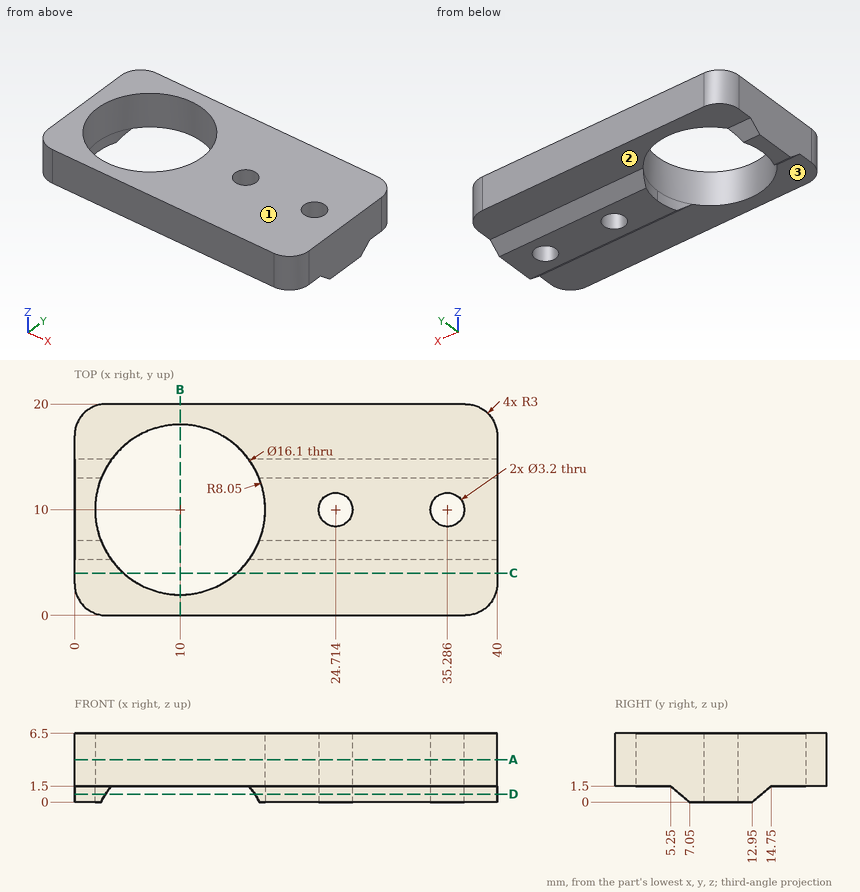
Here's the drawing with two shaded views (mm, measured from the low corner). I have some questions. A direction names the side the tool comes from. Coordinates: 2 decimals unless noted, no trailing zeros. Write each loop counter-clockwise with the first axis right and the second up, starting at its lowest first coordinate (ties: lowest second). Pieces come first, ordered by that corner, then holes. Notation, with made-up numbers: (-13.5, -34.5) -> (28.5, -34.5) arc R27 cw to (28.5, -9.5) -> close; hole circle Ø4 at (-0.5, -32.5). An arc over 180 degrees is marked (long way). Write item = value, one per line. Start each with the question number.
(1) Will these pins go through, and if not, where does the flat tip stop? pin 1 (1.5 mm diameter, centred on y = 9, z = 1.5, fed in from -X); pin 2 (6 mm diameter, centred on x = 10, y = 4, fed in from -Z).
(2) I need wall thicknesses on line 1 (X direction, y = 10, z = 3); line 2 (X direction, y = 9, z = 2) (3 decimals); line 3 (Y direction, x = 10, z = 2.9). Which ranges of each line are inside material? Lowest first, please. Write a range as [from, to].
(3) I want a section at D-D (z = 0.75). Please give me the cut outline in (x, y), plus the area to 3 significant figures.
(4) I want a section at C-C (y = 4). Please give me the cut outline in (x, z), plus the area to 3 significant figures.
(5) Which directions (+Z, -Z, +X, -X, +Y, -Y) give clear straight access to the entire face, cutting with the end or side of a thin tool? Please do the marked faces 1, 2 and 3.
(6) I want a section at B-B (x = 10). Please give me the cut outline in (y, z), plus the area to 3 significant figures.
(7) I want a section at A-A (z = 4). Please give me the cut outline in (x, y).
Result set:
q1.pin_1 = 0
q1.pin_2 = 1.5
q2.line_1 = [0, 1.95], [18.05, 23.11], [26.31, 33.69], [36.89, 40]
q2.line_2 = [0, 2.012], [17.988, 23.465], [25.963, 34.037], [36.535, 40]
q2.line_3 = [0, 1.95], [18.05, 20]
q3.outline = (0, 6.15) -> (2.93, 6.15) arc R8.05 cw to (2.93, 13.85) -> (0, 13.85) -> close; (17.07, 6.15) -> (40, 6.15) -> (40, 13.85) -> (17.07, 13.85) arc R8.05 cw to (18.05, 10) arc R8.05 cw to start; hole circle Ø3.2 at (24.71, 10); hole circle Ø3.2 at (35.29, 10)
q3.area = 173 mm2
q4.outline = (0, 1.5) -> (4.63, 1.5) -> (4.63, 6.5) -> (0, 6.5) -> close; (15.37, 1.5) -> (40, 1.5) -> (40, 6.5) -> (15.37, 6.5) -> close
q4.area = 146 mm2
q5.face_1 = +Z, +X, -X, +Y, -Y
q5.face_2 = -Z, +X, -X, +Y
q5.face_3 = -Z, +X, -X, -Y
q6.outline = (0, 1.5) -> (1.95, 1.5) -> (1.95, 6.5) -> (0, 6.5) -> close; (18.05, 1.5) -> (20, 1.5) -> (20, 6.5) -> (18.05, 6.5) -> close
q6.area = 19.5 mm2
q7.outline = (0, 3) arc R3 ccw to (3, 0) -> (37, 0) arc R3 ccw to (40, 3) -> (40, 17) arc R3 ccw to (37, 20) -> (3, 20) arc R3 ccw to (0, 17) -> close; hole circle Ø16.1 at (10, 10); hole circle Ø3.2 at (24.71, 10); hole circle Ø3.2 at (35.29, 10)
